from build123d import *

# Parameters (mm, degrees)
SKETCH1_R                                  = 40
BOSS_EXTRUDE1_DEPTH                        = 50
SKETCH2_R                                  = 10.425
CUT_EXTRUDE1_DEPTH                         = 30
SKETCH3_R                                  = 20
SKETCH3_R_2                                = 10
CUT_EXTRUDE2_DEPTH                         = 5
SKETCH4_R                                  = 0.5
CUT_EXTRUDE3_DEPTH                         = 76.498344353
SKETCH5_R                                  = 2.5
CUT_EXTRUDE4_DEPTH                         = 76.498344353
CUT_EXTRUDE5_START                         = -49.839677
SKETCH7_R                                  = 1.25
CUT_EXTRUDE5_DEPTH                         = 50.817776
MIRROR1_START                              = -49.839677
MIRROR1_AT_THE_SECOND_PLANE_COPY_1_SKETC_R = 1.25
MIRROR1_AT_THE_SECOND_PLANE_COPY_1_DEPTH   = 50.817776


with BuildPart() as part:
    # Sketch1 → Boss-Extrude1 (new body)
    with BuildSketch(Plane(origin=(0, 0, 0), x_dir=(0, 0, -1), z_dir=(1, 0, 0))):
        Circle(SKETCH1_R)
    extrude(amount=BOSS_EXTRUDE1_DEPTH)

    # Sketch2 → Cut-Extrude1 (cut)
    with BuildSketch(Plane(origin=(50, 0, 0), x_dir=(0, 0, -1), z_dir=(1, 0, 0))):
        Circle(SKETCH2_R)
    extrude(amount=-CUT_EXTRUDE1_DEPTH, mode=Mode.SUBTRACT)

    # Sketch3 → Cut-Extrude2 (cut)
    with BuildSketch(Plane.ZY):
        Circle(SKETCH3_R)
        Circle(SKETCH3_R_2, mode=Mode.SUBTRACT)
    extrude(amount=-CUT_EXTRUDE2_DEPTH, mode=Mode.SUBTRACT)

    # Sketch4 → Cut-Extrude3 (cut, through all)
    with BuildSketch(Plane.ZY):
        Circle(SKETCH4_R)
    extrude(amount=-CUT_EXTRUDE3_DEPTH, mode=Mode.SUBTRACT)

    # Sketch5 → Cut-Extrude4 (cut, through all)
    with BuildSketch(Plane.ZY):
        with Locations((0, 30)):
            Circle(SKETCH5_R)
        with Locations((30, 0)):
            Circle(SKETCH5_R)
        with Locations((0, -30)):
            Circle(SKETCH5_R)
        with Locations((-30, 0)):
            Circle(SKETCH5_R)
    extrude(amount=-CUT_EXTRUDE4_DEPTH, mode=Mode.SUBTRACT)

    # Sketch7 → Cut-Extrude5 (cut)
    with BuildSketch(Plane(origin=(0, 0, 0), x_dir=(0, 0, 1), z_dir=(-0.9063077870366496, 0.42261826174070033, 0)).offset(CUT_EXTRUDE5_START)):
        with Locations(Location((0, 12.678547852, 0), (0, 0, 90))):
            Circle(SKETCH7_R)
    cut_extrude5 = extrude(amount=CUT_EXTRUDE5_DEPTH, mode=Mode.SUBTRACT)

    # Mirror1: Cut-Extrude5 across plane
    add(cut_extrude5.mirror(Plane.ZX), mode=Mode.SUBTRACT)

    # Mirror1 at the second plane: Cut-Extrude5 across plane
    add(cut_extrude5.mirror(Plane.XY), mode=Mode.SUBTRACT)

    # Mirror1 at the second plane copy 1 sketc → Mirror1 at the second plane copy 1 (cut)
    with BuildSketch(Plane(origin=(0, 0, 0), x_dir=(0, 0, -1), z_dir=(-0.9063077870366496, -0.42261826174070033, 0)).offset(MIRROR1_START)):
        with Locations(Location((0, 12.678547852, 0), (0, 0, 90))):
            Circle(MIRROR1_AT_THE_SECOND_PLANE_COPY_1_SKETC_R)
    extrude(amount=MIRROR1_AT_THE_SECOND_PLANE_COPY_1_DEPTH, mode=Mode.SUBTRACT)


solid = part.part
Input: part model. Units: mm. Frame: model coordinates. A direction names the side the tool comes from. Round coordinates to 2 decimals unless told otherwise and drop trailing zeros. Order: outer loops, then holes, each group sorted by start corner. A loop starts at its lowest first (then second) coordinate and runs counter-clockwise, first axis right, second up. Notation, with made-up numbers: (2, -21.5) - (40, -21.5) arc R36 ccw to (40, 14.5) - close; hole circle Ø6 at (9, 37.25). An arc over 180 degrees is marked (long way). Use a Markdown table: item, result.
1. Section D-D on x = 46.5. Return the cut outline in (y, z) (3 decimals).
Evaluation:
| item | result |
|---|---|
| outline | circle Ø80 at (0, 0); hole circle Ø5 at (-30, 0); hole circle Ø20.85 at (0, 0); hole circle Ø5 at (0, -30); hole circle Ø5 at (0, 30); hole circle Ø5 at (30, 0) |
2. Material intervals for probe 1 along Y at (x, z) = (4.05, 0); probe 2 along Y at (x, z) = (20.5, 0) (3 decimals); probe 3 along Z at (x, y) = (36.5, 1.5), sorted ascending.
Evaluation:
| item | result |
|---|---|
| probe 1 | -40 to -32.5, -27.5 to -20, -10 to -0.5, 0.5 to 10, 20 to 27.5, 32.5 to 40 |
| probe 2 | -40 to -32.5, -27.5 to -10.425, 10.425 to 27.5, 32.5 to 40 |
| probe 3 | -39.97 to -32, -28 to -10.32, 10.32 to 28, 32 to 39.97 |
3. Access query for faces 1 (the face through (20, -2, 0)), 2 (the face through (24.6, 0.1, 27.5)), 3 (the face through (2.465, -19.524, -4.336)). Directions: +Z, -Z, +X, -X, +Y, -Y. A direction counts if a zero-diameter tool reaches every point of the face in a straight line with its end or side. Return the directions, or none.
Evaluation:
| item | result |
|---|---|
| face 1 | +X |
| face 2 | +X, -X |
| face 3 | -X |
4. Mould query, pull axis Y, two halves, no side actions, for faces 4 (the face through (0, 0, -2)), 5 (the face through (24.65, -39.05, 8.67)), 6 (the face through (12.11, 6.964, -0.055)). Classes: +Y half, -Y half, draft (parallel to the pull), parting line (faces both ways), or undercut.
Evaluation:
| item | result |
|---|---|
| face 4 | draft |
| face 5 | parting line |
| face 6 | undercut |
5. Section B-B on y = 30. Return the cut outline in (x, z).
Evaluation:
| item | result |
|---|---|
| outline | (0, -26.46) - (50, -26.46) - (50, -2.5) - (0, -2.5) - close; (0, 2.5) - (50, 2.5) - (50, 26.46) - (0, 26.46) - close |
6. Section A-A on x = 3.5. Return the cut outline in (y, z).
Evaluation:
| item | result |
|---|---|
| outline | circle Ø80 at (0, 0); circle Ø20 at (0, 0); hole circle Ø5 at (-30, 0); hole circle Ø40 at (0, 0); hole circle Ø5 at (0, -30); hole circle Ø5 at (0, 30); hole circle Ø1 at (0, 0); hole circle Ø5 at (30, 0) |
7. First-contact query: pin 1 (6 mm diameter, centred on x = 32.5, z = 5, fed in from +Y); pin 2 (2 mm diameter, centred on x = 40.5, y = 13.5, fed in from -Z); pin 3 (5 mm diameter, centred on x = 40.5, z = -3.5, fed in from +Y); pin 4 (3 mm diameter, centred on y = -30, z = 0, fed in from +X). Flat tips, straight axial feed; report the tip coordinate or a pass-through.
Evaluation:
| item | result |
|---|---|
| pin 1 | y = 39.95 |
| pin 2 | z = -38 |
| pin 3 | y = 39.99 |
| pin 4 | through |
